Design review of the part shown in the three views and the two pictorial views. Dimensions are in mm from the part's minimum x, y and z. Coordinates: 2 decimals unless noted, no trailing zeros. Loops run counter-clockwise (first coordinate to the right, second up) from the corner with the lowest first, then second, coordinate; pieces in that order, holes last. Notation, with made-up numbers: M -3,-34.75 L 1,-34.75 A31 cw 1,0.25 Z; hole C 55.5,57.25 d6. An arc over 180 degrees is marked long. Put each result on its own line as item: value. Start each with the question number.
(1) Take a section at D-D, the plane x = 10. Give the boundary of the cut face in (y, z).
(2) Take a section at B-B, the plane y = 14.75. Give the boundary of the cut face in (x, z).
(3) The part is to be moulded in two halves that separate along X. For the marked faces 1, 2, 3 and 4, say which applies: +X half, -X half, draft (parallel to the pull), parting line (faces both ways), or undercut.
(4) Take a section at C-C, the plane z = 7. Give the boundary of the cut face in (x, y).
(5) For probe 1 along X at (y, z) = (4, 1); probe 2 along X at (y, z) = (19, 9.5); probe 3 along Z at (x, y) = (10, 14), list the stretches that pass through material, from the lowest coordinate up. Write a range as [from, to].
(6) Take a section at A-A, the plane z = 3. Give the boundary of the cut face in (x, y).
(7) Clearance check with a flat-ended pin moving along its axis: pin 1 (6 mm diameter, centred on x = 10.5, y = 4.5, fed in from -Z). State where the tip first meets the part, or that it passes through.
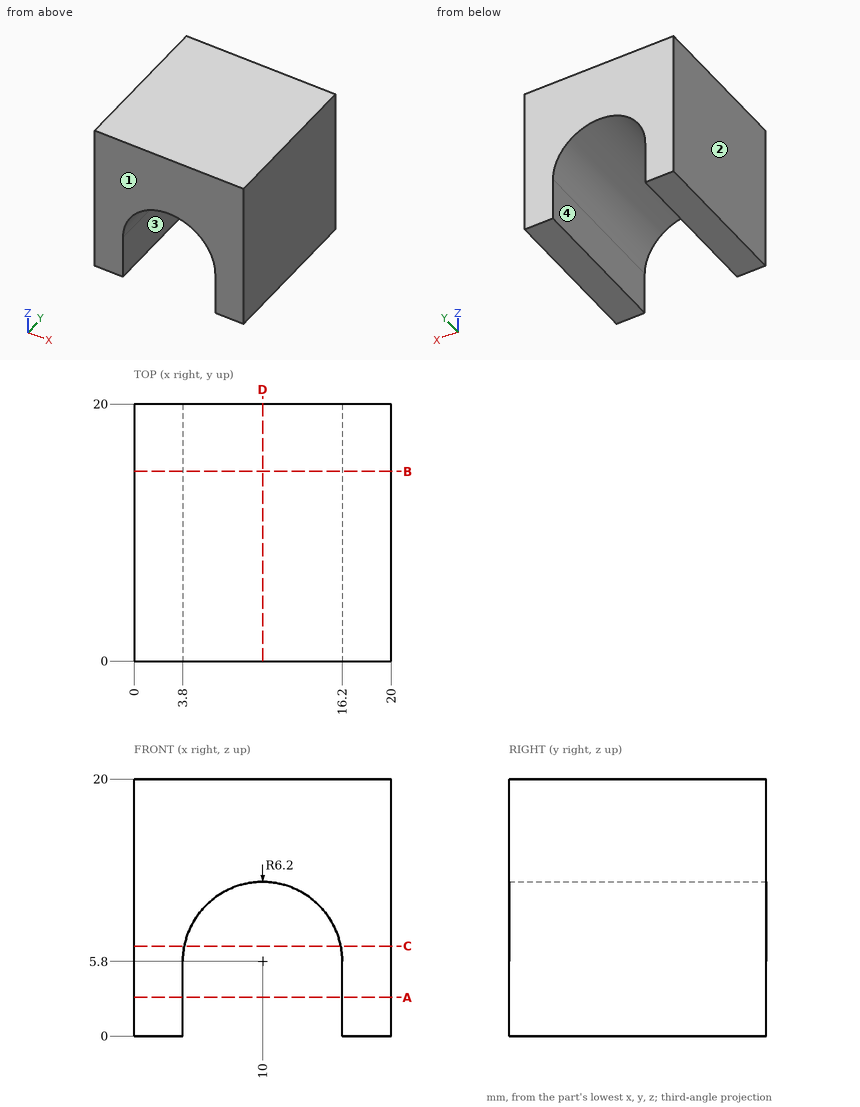
Computed values:
1. outline: M 0,12 L 20,12 L 20,20 L 0,20 Z
2. outline: M 0,0 L 3.8,0 L 3.8,5.8 A6.2 cw 16.2,5.8 L 16.2,0 L 20,0 L 20,20 L 0,20 Z
3. face 1: draft
3. face 2: -X half
3. face 3: undercut
3. face 4: undercut
4. outline: M 0,0 L 3.92,0 L 3.92,20 L 0,20 Z; M 16.08,0 L 20,0 L 20,20 L 16.08,20 Z
5. probe 1: x = [0, 3.8], [16.2, 20]
5. probe 2: x = [0, 5.03], [14.97, 20]
5. probe 3: z = [12, 20]
6. outline: M 0,0 L 3.8,0 L 3.8,20 L 0,20 Z; M 16.2,0 L 20,0 L 20,20 L 16.2,20 Z
7. pin 1: stops at z = 10.92
